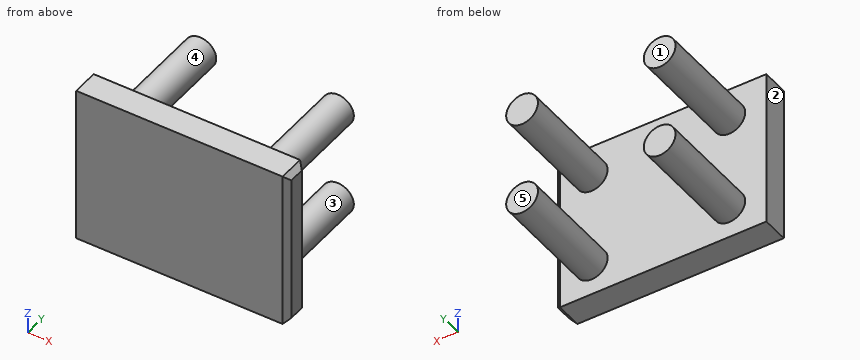
```python
from build123d import *

# Parameters (mm, degrees)
F0_W     = 80
F0_H     = 60
F1_DEPTH = 10
F2_R     = 6
F3_DEPTH = 40
F4_SIZE  = 2


with BuildPart() as f1:
    # F0 (on Front) → F1 (new body)
    with BuildSketch(Plane.XZ):
        Rectangle(F0_W, F0_H)
    extrude(amount=F1_DEPTH)

    # F2 (on face) → F3 (join)
    with BuildSketch(Plane(origin=(0, 0, 0), x_dir=(-1, 0, 0), z_dir=(0, 1, 0))):
        with Locations((26, 18)):
            Circle(F2_R)
        with Locations((26, -18)):
            Circle(F2_R)
        with Locations((-26, -18)):
            Circle(F2_R)
        with Locations((-26, 18)):
            Circle(F2_R)
    extrude(amount=F3_DEPTH)

    # F4
    f4_edges = [f1.edges().sort_by_distance(p)[0] for p in [
        (40, -5, -30),
        (40, -5, 30),
        (40, 0, 0),
        (40, -10, 0),
    ]]
    chamfer(f4_edges, length=F4_SIZE)


solid = f1.part
```
Read the model definition and answer for the solid it produces. Units are mm, in the model's axes. Face numbers are marked on the shaded views. A direction names the side the tool comes from. Give positions to 0.01 mm unless a question says otherwise; leave off trailing zeros. Order: outer loops, then holes, each group sorted by start corner. A loop starts at its lowest first (then second) coordinate and runs counter-clockwise, first axis right, second up.
(1) Find section B-B (z = 18). Give the vertices of the cut face in (x, y).
(2) Find section A-A (x = 26). Give the vertices of the cut face in (y, z).
(3) Given pin 1 (18 mm diameter, centred on x = -3, z = -7.5, fed in from +Y); pin 2 (1 mm diameter, centred on x = -22, y = 13.5, fed in from +Z); pin 3 (8 mm diameter, centred on y = 34, z = -23, fed in from -X), each flat-ended and moving along its own axis, determine where each tip first touches the part or whether it passes through.
(4) Find section D-D (x = -21). Give the vertices of the cut face in (y, z), plus the area to 3 significant figures.
(5) Straight lines are drawn through the part: L1, parallel to Z at x = -26, y = 15; L2, parallel to Y at x = -16, z = 7; L3, parallel to X at y = 13.5, z = 14.5. For each, find the intervals that lie inside material, in ascending order.
(6) For a pull along X with two mould halves and no side action, classify the marked faces 1, 2 and 3 as released by +X, released by -X, zero draft, split by the parting line, or undercut.
(7) Find section C-C (y = 14). Give the vertices of the cut face in (x, z).
(8) For the marked faces 4 and 5, determine the directions among +Z, -Z, +X, -X, +Y, -Y from which every point of the face is accessible in a straight line to the end or side of a thin tool.
Result sheet:
1. outline: (-40, -10) - (38, -10) - (40, -8) - (40, -2) - (38, 0) - (32, 0) - (32, 40) - (20, 40) - (20, 0) - (-20, 0) - (-20, 40) - (-32, 40) - (-32, 0) - (-40, 0) - close
2. outline: (-10, -30) - (0, -30) - (0, -24) - (40, -24) - (40, -12) - (0, -12) - (0, 12) - (40, 12) - (40, 24) - (0, 24) - (0, 30) - (-10, 30) - close
3. pin 1: stops at y = 0
3. pin 2: stops at z = 22.87
3. pin 3: stops at x = -31.92
4. outline: (-10, -30) - (0, -30) - (0, -21.32) - (40, -21.32) - (40, -14.68) - (0, -14.68) - (0, 14.68) - (40, 14.68) - (40, 21.32) - (0, 21.32) - (0, 30) - (-10, 30) - close
4. area: 1,130 mm2
5. L1: z = -24 to -12, 12 to 24
5. L2: y = -10 to 0
5. L3: x = -30.87 to -21.13, 21.13 to 30.87
6. face 1: zero draft
6. face 2: released by -X
6. face 3: undercut
7. outline: circle Ø12 at (-26, -18); circle Ø12 at (-26, 18); circle Ø12 at (26, -18); circle Ø12 at (26, 18)
8. face 4: +Y
8. face 5: +Z, -Z, +X, -X, +Y
